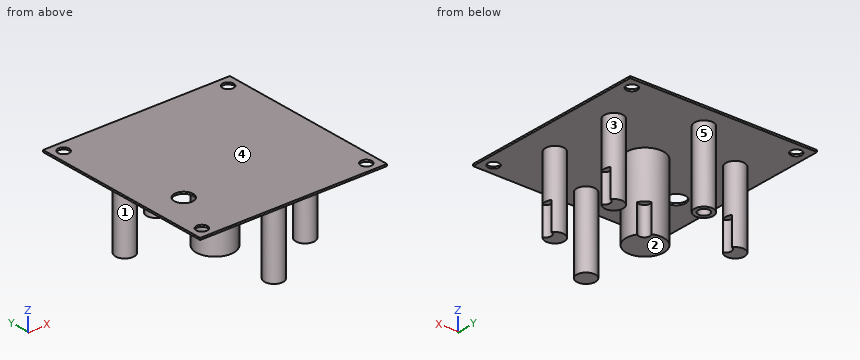
```python
from build123d import *

# Parameters (mm, degrees)
SKETCH001_W       = 200
SKETCH001_H       = 200
SKETCH001_R       = 6
SKETCH001_R_2     = 10
SKETCH001_R_3     = 20
PAD_DEPTH         = 2
SKETCH_R          = 10
SKETCH_R_2        = 20
PAD001_DEPTH      = 80
PAD001_DEPTH_BACK = 2
SKETCH002_R       = 6
POCKET_DEPTH      = 30


with BuildPart() as part:
    # Sketch001 → Pad (new body)
    with BuildSketch(Plane.XY):
        with Locations((100, 100)):
            Rectangle(SKETCH001_W, SKETCH001_H)
        with Locations((12, 12)):
            Circle(SKETCH001_R, mode=Mode.SUBTRACT)
        with Locations((12, 188)):
            Circle(SKETCH001_R, mode=Mode.SUBTRACT)
        with Locations((188, 188)):
            Circle(SKETCH001_R, mode=Mode.SUBTRACT)
        with Locations((188, 12)):
            Circle(SKETCH001_R, mode=Mode.SUBTRACT)
        with Locations((100, 175)):
            Circle(SKETCH001_R_2, mode=Mode.SUBTRACT)
        with Locations((35.048095, 137.5)):
            Circle(SKETCH001_R_2, mode=Mode.SUBTRACT)
        with Locations((35.048095, 62.5)):
            Circle(SKETCH001_R_2, mode=Mode.SUBTRACT)
        with Locations((100, 25)):
            Circle(SKETCH001_R_2, mode=Mode.SUBTRACT)
        with Locations((164.951905, 62.5)):
            Circle(SKETCH001_R_2, mode=Mode.SUBTRACT)
        with Locations((164.951905, 137.5)):
            Circle(SKETCH001_R_2, mode=Mode.SUBTRACT)
        with Locations((100, 100)):
            Circle(SKETCH001_R_3, mode=Mode.SUBTRACT)
    extrude(amount=PAD_DEPTH)

    # Sketch (on Face16 of Pad) → Pad001 (new body, two sides)
    with BuildSketch(Plane(origin=(0, 0, 0), x_dir=(1, 0, 0), z_dir=(0, 0, -1))) as pad001_sk:
        with Locations((164.951905, -62.5)):
            Circle(SKETCH_R)
        with Locations((100, -175)):
            Circle(SKETCH_R)
        with Locations((100, -25)):
            Circle(SKETCH_R)
        with Locations((35.048095, -137.5)):
            Circle(SKETCH_R)
        with Locations((164.951905, -137.5)):
            Circle(SKETCH_R)
        with Locations((100, -100)):
            Circle(SKETCH_R_2)
    extrude(amount=PAD001_DEPTH)
    extrude(pad001_sk.sketch, amount=-PAD001_DEPTH_BACK)

    # Sketch002 (on Face24 of Pad001) → Pocket (cut)
    with BuildSketch(Plane(origin=(0, 0, -80), x_dir=(1, 0, 0), z_dir=(0, 0, -1))):
        with Locations((113.064442, -114.794754)):
            Circle(SKETCH002_R)
        with Locations((35.048095, -62.5)):
            Circle(SKETCH002_R)
        with Locations((100, -175)):
            Circle(SKETCH002_R)
        with Locations((45.048095, -137.5)):
            Circle(SKETCH002_R)
        with Locations((174.951905, -62.5)):
            Circle(SKETCH002_R)
        with Locations((174.951905, -137.5)):
            Circle(SKETCH002_R)
    extrude(amount=-POCKET_DEPTH, mode=Mode.SUBTRACT)


solid = part.part
```
Build history of the part. All positions in model axes, mm. Face numbers are marked on the shaded views. A direction names the side the tool comes from. Coordinates: 2 decimals unless noted, no trailing zeros. Order: outer loops, then holes, each group sorted by start corner. A loop starts at its lowest first (then second) coordinate and runs counter-clockwise, first axis right, second up. Notation, with made-up numbers: (-15.75, 81.25) -> (14.25, 81.25) arc R35 ccw to (14.25, 113.25) -> close; hole circle Ø3 at (-4.5, 73). An arc over 180 degrees is marked (long way). Answer in a Markdown table with one row per item. Add a question column.
Q1. Band-saw the part on D-D, the plane z = -65. List the corners of the cut face in (x, y), then the cut area to 3 significant figures.
Q2. Wall check: line 1 along Y through (x, z) = (100, -65.75); line 2 along Y through (x, z) = (188, 0.9); line 3 along Z through (x, y) = (112, 62). Give the ranges that are in metal, low to high. Write a range as [from, to].
Q3. Band-saw the part on A-A, the plane y = 12. List the corners of the cut face in (x, z).
Q4. Drop flat-ended pins along their axis: pin 1 (7.5 mm diameter, centred on x = 111.5, y = 114, fed in from -Z); pin 2 (15.5 mm diameter, centred on x = 12, y = 188, fed in from -Z); pin 3 (12 mm diameter, centred on y = 126.5, z = -33, fed in from -X). Give the stop position or say it passes through.
Q5. Which spindle directions (+Z, -Z, +X, -X, +Y, -Y) get a long thin tool onto all of the face, cutting with end or side? Do the marked faces 1 and 2. Say none if no direction does.
Q6. Mould opens along X. For the marked faces 3, 4 and 5 say: +X half, -X half, draft (parallel to the pull), parting line (faces both ways), or undercut.
Q7. Band-saw the part on C-C, the plane z = -24. List the corners of the cut face in (x, y), then the cut area to 3 significant figures.
Answers follow:
| question | item | result |
|---|---|---|
| 1 | outline | (43.25, 131.78) arc R6 cw to (43.25, 143.22) arc R10 ccw (long way) to start; circle Ø20 at (100, 25); circle Ø20 at (100, 175); (108.16, 118.26) arc R20 ccw (long way) to (117.11, 110.36) arc R6 cw to start; (173.15, 56.78) arc R6 cw to (173.15, 68.22) arc R10 ccw (long way) to start; (173.15, 131.78) arc R6 cw to (173.15, 143.22) arc R10 ccw (long way) to start; hole circle Ø12 at (100, 175) |
| 1 | area | 2,510 mm^2 |
| 2 | line 1 | [15, 35], [80, 120], [165, 169], [181, 185] |
| 2 | line 2 | [0, 6], [18, 182], [194, 200] |
| 2 | line 3 | [0, 2] |
| 3 | outline | (0, 0) -> (6, 0) -> (6, 2) -> (0, 2) -> close; (18, 0) -> (182, 0) -> (182, 2) -> (18, 2) -> close; (194, 0) -> (200, 0) -> (200, 2) -> (194, 2) -> close |
| 4 | pin 1 | z = -50 |
| 4 | pin 2 | z = 0 |
| 4 | pin 3 | x = 26.39 |
| 5 | face 1 | -Z |
| 5 | face 2 | -Z, +X, -X, +Y, -Y |
| 6 | face 3 | undercut |
| 6 | face 4 | draft |
| 6 | face 5 | parting line |
| 7 | outline | circle Ø20 at (35.05, 137.5); circle Ø40 at (100, 100); circle Ø20 at (100, 25); circle Ø20 at (100, 175); circle Ø20 at (164.95, 62.5); circle Ø20 at (164.95, 137.5) |
| 7 | area | 2,830 mm^2 |
